Could you check a few things on this model? Use its own coordinates, in mm. A direction names the side the tool comes from. Round coordinates to 2 decimals unless told otherwise and drop trailing zeros. Write each loop counter-clockwise with the first axis right and the second up, starting at its lowest first coordinate (ties: lowest second). Pieces come first, ordered by that corner, then holes. Notation, with made-up numbers: (56, -4) -> (61, -4) arc R11 cw to (61, 14) -> close; hole circle Ø10 at (19.25, 64). An arc over 180 degrees is marked (long way). Answer in a Markdown table with one row per item.
from build123d import *

# Parameters (mm, degrees)
F0_W     = 115
F0_H     = 39
F1_DEPTH = 8.5
F2_R     = 10
F2_R_2   = 2.525
F3_DEPTH = 2.5
F4_R     = 2.575
F5_DEPTH = 115.001
F7_DEPTH = 5
F8_R     = 8.05
F9_DEPTH = 5


with BuildPart() as f1:
    # F0 (on Top) → F1 (new body)
    with BuildSketch(Plane.XY):
        Rectangle(F0_W, F0_H)
    extrude(amount=F1_DEPTH)

    # F2 (on face) → F3 (join)
    with BuildSketch(Plane(origin=(-57.5, 0, 0), x_dir=(0, -1, 0), z_dir=(-1, 0, 0))):
        with Locations((0, 4.25)):
            Circle(F2_R)
        with Locations((0, 4.25)):
            Circle(F2_R_2, mode=Mode.SUBTRACT)
    extrude(amount=F3_DEPTH)

    # F4 (on face) → F5 (cut, through all)
    with BuildSketch(Plane(origin=(-57.5, 0, 0), x_dir=(0, -1, 0), z_dir=(-1, 0, 0))):
        with Locations((0, 4.4)):
            Circle(F4_R)
    extrude(amount=-F5_DEPTH, mode=Mode.SUBTRACT)

    # F6 (on face) → F7 (join)
    with BuildSketch(Plane(origin=(-60, 0, 0), x_dir=(0, -1, 0), z_dir=(-1, 0, 0))):
        with BuildLine():
            ThreePointArc((0.518394, 16.889246), (0, 16.9), (-0.518394, 16.889246))
            Line((-0.518394, 16.889246), (-1, 15.856439))
            Line((-1, 15.856439), (-1, 14.496058))
            ThreePointArc((-1, 14.496058), (-1.5871, 14.420554), (-2.168797, 14.310939))
            Line((-2.168797, 14.310939), (-2.589178, 15.604738))
            Line((-2.589178, 15.604738), (-3.366367, 16.438171))
            ThreePointArc((-3.366367, 16.438171), (-3.862712, 16.288206), (-4.352412, 16.117786))
            Line((-4.352412, 16.117786), (-4.491291, 14.986704))
            Line((-4.491291, 14.986704), (-4.07091, 13.692905))
            ThreePointArc((-4.07091, 13.692905), (-4.605943, 13.439672), (-5.125297, 13.155668))
            Line((-5.125297, 13.155668), (-5.924909, 14.256239))
            Line((-5.924909, 14.256239), (-6.921605, 14.808717))
            ThreePointArc((-6.921605, 14.808717), (-7.347316, 14.512712), (-7.760384, 14.199308))
            Line((-7.760384, 14.199308), (-7.542943, 13.080669))
            Line((-7.542943, 13.080669), (-6.743331, 11.980097))
            ThreePointArc((-6.743331, 11.980097), (-7.173924, 11.573924), (-7.580097, 11.143331))
            Line((-7.580097, 11.143331), (-8.680669, 11.942943))
            Line((-8.680669, 11.942943), (-9.799308, 12.160384))
            ThreePointArc((-9.799308, 12.160384), (-10.112712, 11.747316), (-10.408717, 11.321605))
            Line((-10.408717, 11.321605), (-9.856239, 10.324909))
            Line((-9.856239, 10.324909), (-8.755668, 9.525297))
            ThreePointArc((-8.755668, 9.525297), (-9.039672, 9.005943), (-9.292905, 8.47091))
            Line((-9.292905, 8.47091), (-10.586704, 8.891291))
            Line((-10.586704, 8.891291), (-11.717786, 8.752412))
            ThreePointArc((-11.717786, 8.752412), (-11.888206, 8.262712), (-12.038171, 7.766367))
            Line((-12.038171, 7.766367), (-11.204738, 6.989178))
            Line((-11.204738, 6.989178), (-9.910939, 6.568797))
            ThreePointArc((-9.910939, 6.568797), (-10.020554, 5.9871), (-10.096058, 5.4))
            Line((-10.096058, 5.4), (-11.456439, 5.4))
            Line((-11.456439, 5.4), (-12.489246, 4.918394))
            ThreePointArc((-12.489246, 4.918394), (-12.5, 4.4), (-12.489246, 3.881606))
            Line((-12.489246, 3.881606), (-11.456439, 3.4))
            Line((-11.456439, 3.4), (-10.096058, 3.4))
            ThreePointArc((-10.096058, 3.4), (-10.020554, 2.8129), (-9.910939, 2.231203))
            Line((-9.910939, 2.231203), (-11.204738, 1.810822))
            Line((-11.204738, 1.810822), (-12.038171, 1.033633))
            ThreePointArc((-12.038171, 1.033633), (-11.888206, 0.537288), (-11.717786, 0.047588))
            Line((-11.717786, 0.047588), (-10.586704, -0.091291))
            Line((-10.586704, -0.091291), (-9.292905, 0.32909))
            ThreePointArc((-9.292905, 0.32909), (-9.039672, -0.205943), (-8.755668, -0.725297))
            Line((-8.755668, -0.725297), (-9.856239, -1.524909))
            Line((-9.856239, -1.524909), (-10.408717, -2.521605))
            ThreePointArc((-10.408717, -2.521605), (-10.112712, -2.947316), (-9.799308, -3.360384))
            Line((-9.799308, -3.360384), (-8.680669, -3.142943))
            Line((-8.680669, -3.142943), (-7.580097, -2.343331))
            ThreePointArc((-7.580097, -2.343331), (-7.173924, -2.773924), (-6.743331, -3.180097))
            Line((-6.743331, -3.180097), (-7.542943, -4.280669))
            Line((-7.542943, -4.280669), (-7.760384, -5.399308))
            ThreePointArc((-7.760384, -5.399308), (-7.347316, -5.712712), (-6.921605, -6.008717))
            Line((-6.921605, -6.008717), (-5.924909, -5.456239))
            Line((-5.924909, -5.456239), (-5.125297, -4.355668))
            ThreePointArc((-5.125297, -4.355668), (-4.605943, -4.639672), (-4.07091, -4.892905))
            Line((-4.07091, -4.892905), (-4.491291, -6.186704))
            Line((-4.491291, -6.186704), (-4.352412, -7.317786))
            ThreePointArc((-4.352412, -7.317786), (-3.862712, -7.488206), (-3.366367, -7.638171))
            Line((-3.366367, -7.638171), (-2.589178, -6.804738))
            Line((-2.589178, -6.804738), (-2.168797, -5.510939))
            ThreePointArc((-2.168797, -5.510939), (-1.5871, -5.620554), (-1, -5.696058))
            Line((-1, -5.696058), (-1, -7.056439))
            Line((-1, -7.056439), (-0.518394, -8.089246))
            ThreePointArc((-0.518394, -8.089246), (0, -8.1), (0.518394, -8.089246))
            Line((0.518394, -8.089246), (1, -7.056439))
            Line((1, -7.056439), (1, -5.696058))
            ThreePointArc((1, -5.696058), (1.5871, -5.620554), (2.168797, -5.510939))
            Line((2.168797, -5.510939), (2.589178, -6.804738))
            Line((2.589178, -6.804738), (3.366367, -7.638171))
            ThreePointArc((3.366367, -7.638171), (3.862712, -7.488206), (4.352412, -7.317786))
            Line((4.352412, -7.317786), (4.491291, -6.186704))
            Line((4.491291, -6.186704), (4.07091, -4.892905))
            ThreePointArc((4.07091, -4.892905), (4.605943, -4.639672), (5.125297, -4.355668))
            Line((5.125297, -4.355668), (5.924909, -5.456239))
            Line((5.924909, -5.456239), (6.921605, -6.008717))
            ThreePointArc((6.921605, -6.008717), (7.347316, -5.712712), (7.760384, -5.399308))
            Line((7.760384, -5.399308), (7.542943, -4.280669))
            Line((7.542943, -4.280669), (6.743331, -3.180097))
            ThreePointArc((6.743331, -3.180097), (7.173924, -2.773924), (7.580097, -2.343331))
            Line((7.580097, -2.343331), (8.680669, -3.142943))
            Line((8.680669, -3.142943), (9.799308, -3.360384))
            ThreePointArc((9.799308, -3.360384), (10.112712, -2.947316), (10.408717, -2.521605))
            Line((10.408717, -2.521605), (9.856239, -1.524909))
            Line((9.856239, -1.524909), (8.755668, -0.725297))
            ThreePointArc((8.755668, -0.725297), (9.039672, -0.205943), (9.292905, 0.32909))
            Line((9.292905, 0.32909), (10.586704, -0.091291))
            Line((10.586704, -0.091291), (11.717786, 0.047588))
            ThreePointArc((11.717786, 0.047588), (11.888206, 0.537288), (12.038171, 1.033633))
            Line((12.038171, 1.033633), (11.204738, 1.810822))
            Line((11.204738, 1.810822), (9.910939, 2.231203))
            ThreePointArc((9.910939, 2.231203), (10.020554, 2.8129), (10.096058, 3.4))
            Line((10.096058, 3.4), (11.456439, 3.4))
            Line((11.456439, 3.4), (12.489246, 3.881606))
            ThreePointArc((12.489246, 3.881606), (12.5, 4.4), (12.489246, 4.918394))
            Line((12.489246, 4.918394), (11.456439, 5.4))
            Line((11.456439, 5.4), (10.096058, 5.4))
            ThreePointArc((10.096058, 5.4), (10.020554, 5.9871), (9.910939, 6.568797))
            Line((9.910939, 6.568797), (11.204738, 6.989178))
            Line((11.204738, 6.989178), (12.038171, 7.766367))
            ThreePointArc((12.038171, 7.766367), (11.888206, 8.262712), (11.717786, 8.752412))
            Line((11.717786, 8.752412), (10.586704, 8.891291))
            Line((10.586704, 8.891291), (9.292905, 8.47091))
            ThreePointArc((9.292905, 8.47091), (9.039672, 9.005943), (8.755668, 9.525297))
            Line((8.755668, 9.525297), (9.856239, 10.324909))
            Line((9.856239, 10.324909), (10.408717, 11.321605))
            ThreePointArc((10.408717, 11.321605), (10.112712, 11.747316), (9.799308, 12.160384))
            Line((9.799308, 12.160384), (8.680669, 11.942943))
            Line((8.680669, 11.942943), (7.580097, 11.143331))
            ThreePointArc((7.580097, 11.143331), (7.173924, 11.573924), (6.743331, 11.980097))
            Line((6.743331, 11.980097), (7.542943, 13.080669))
            Line((7.542943, 13.080669), (7.760384, 14.199308))
            ThreePointArc((7.760384, 14.199308), (7.347316, 14.512712), (6.921605, 14.808717))
            Line((6.921605, 14.808717), (5.924909, 14.256239))
            Line((5.924909, 14.256239), (5.125297, 13.155668))
            ThreePointArc((5.125297, 13.155668), (4.605943, 13.439672), (4.07091, 13.692905))
            Line((4.07091, 13.692905), (4.491291, 14.986704))
            Line((4.491291, 14.986704), (4.352412, 16.117786))
            ThreePointArc((4.352412, 16.117786), (3.862712, 16.288206), (3.366367, 16.438171))
            Line((3.366367, 16.438171), (2.589178, 15.604738))
            Line((2.589178, 15.604738), (2.168797, 14.310939))
            ThreePointArc((2.168797, 14.310939), (1.5871, 14.420554), (1, 14.496058))
            Line((1, 14.496058), (1, 15.856439))
            Line((1, 15.856439), (0.518394, 16.889246))
        make_face()
    extrude(amount=F7_DEPTH)

    # F8 (on face) → F9 (cut)
    with BuildSketch(Plane(origin=(-65, 0, 0), x_dir=(0, -1, 0), z_dir=(-1, 0, 0))):
        with Locations((0, 4.4)):
            Circle(F8_R)
    extrude(amount=-F9_DEPTH, mode=Mode.SUBTRACT)


solid = f1.part
1) Imagine slicing it at A-A, the plane x = -2. Please give me the cut outline in (y, z) (3 decimals).
Findings:
| item | result |
|---|---|
| outline | (-19.5, 0) -> (19.5, 0) -> (19.5, 8.5) -> (-19.5, 8.5) -> close; hole circle Ø5.15 at (0, 4.4) |
2) For pin 1 (4.5 mm diameter, centred on y = 0, z = 4.4, fed in from -X); pin 2 (12 mm diameter, centred on x = 9, y = 5.5, fed in from +Z); pin 3 (4 mm diameter, centred on y = -15, z = 4.5, fed in from -X); pin 4 (10 mm diameter, centred on x = -19, y = 3.5, fed in from -Z), each with a flat end and sliding along its axis, tell me the tip position at first contact or that it passes through.
Findings:
| item | result |
|---|---|
| pin 1 | passes through |
| pin 2 | stops at z = 8.5 |
| pin 3 | stops at x = -57.5 |
| pin 4 | stops at z = 0 |
3) Thinking about a two-plate mould opening in Y: for faces 1 (the face through (-1, -19.5, 4)), 2 (the face through (-57.5, 0, -2)), 3 (the face through (-0.805, -2.456, 5.173)), 4 (the face through (-1, 19.5, 4)), which applies, +Y half, -Y half, draft (parallel to the pull), parting line (faces both ways), or undercut?
Findings:
| item | result |
|---|---|
| face 1 | -Y half |
| face 2 | draft |
| face 3 | undercut |
| face 4 | +Y half |
4) For faces 5 (the face through (57.5, 0, 1)), 6 (the face through (-62.535, 1.745, -3.459)), 7 (the face through (-1, 0, 0)), 8 (the face through (-1, 0, 8.5)), 9 (the face through (-58.732, 1.302, 14.165)), which set-ups out of +Z, -Z, +X, -X, +Y, -Y let a thin tool reach every point of the face, with its end or its side?
Findings:
| item | result |
|---|---|
| face 5 | +Z, -Z, +X, +Y, -Y |
| face 6 | -X |
| face 7 | -Z, +X, +Y, -Y |
| face 8 | +Z, +X, +Y, -Y |
| face 9 | none |
5) Please list where these lines run through material, in increasing order: line 1 (Y direction, x = 29, z = 4.5); line 2 (Z direction, x = -59, y = 0) (3 decimals); line 3 (Z direction, x = -63, y = 0).
Findings:
| item | result |
|---|---|
| line 1 | y = -19.5 to -2.57, 2.57 to 19.5 |
| line 2 | z = -5.75 to 1.725, 6.775 to 14.25 |
| line 3 | z = -8.1 to -3.65, 12.45 to 16.9 |
